Can you work these out from the model? Positions are in its coordinate system, mm. A direction names the side the tool comes from. Round coordinates to 2 decimals unless told otherwise and drop trailing zeros. Order: outer loops, then holes, each group sorted by start corner. A loop starts at its lowest first (then second) coordinate and runs counter-clockwise, first axis right, second up.
Q1. For faces 5 (the face through (18.288, -19, 13)), 6 (the face through (105, -20.32, 13)), which set-ups out of +Z, -Z, +X, -X, +Y, -Y let a thin tool reach every point of the face, with its end or its side?
Q2. If we section it at A-A (y = -14): Count the separate pieces of the cut face and the enclosed holes in it, plus the area to 3 significant figures.
Q3. If we section it at C-C (x = 53.5): Please give me the cut outline in (y, z).
Q4. Will this pin go through, and if not, where does the flat tip stop? P1, Ø10, axis at x = 89, z = 21, coming from the -Y side.
Q5. If I drill on line 1 (X direction, y = -15.75, z = 7.5); line 2 (X direction, y = -13.5, z = 14.75); line 3 (Y direction, x = 55, z = 6.75), over which ranges is the centre line in solid material (lowest first)?
Q6. We'd pull the mould along X, two halves only. Please class faces 1 (the face through (58, -8, 25.4)), 2 (the face through (33.25, -16.51, 12.52)), 3 (the face through (96.012, -19, 13)), 4 (the face through (114.3, -10, 13)): pulls with the +X half, pulls with the -X half, needs draft (parallel to the pull), parting line crosses it, or undercut.
Q7. If we section it at B-B (x = 71): Please give me the cut outline in (y, z).
from build123d import *

# Parameters (mm, degrees)
F1_DEPTH = 25.4


with BuildPart() as f1:
    # F0 (on Top) → F1 (new body)
    with BuildSketch(Plane.XY):
        with BuildLine():
            Line((57.15, 0), (0, 0))
            Line((0, 0), (0, -20.32))
            Line((0, -20.32), (18.288, -20.32))
            Line((18.288, -20.32), (18.288, -17.78))
            add(Edge.make_bspline(
                [(18.288, -17.78), (19.5003372633, -17.78), (20.9589545485, -17.4917433662), (23.0646434791, -15.3048474183), (24.9900381466, -13.3300613523), (27.3662145743, -12.7), (28.575, -12.7)],
                knots=[0, 0, 0, 0, 0.2397485597, 0.4832453932, 0.7259444723, 1, 1, 1, 1], degree=3))
            ThreePointArc((28.575, -12.7), (33.3375, -16.51), (38.1, -12.7))
            ThreePointArc((38.1, -12.7), (47.2236683009, -16.8621762468), (57.15, -18.288))
            Line((57.15, -18.288), (57.15, 0))
        make_face()
    extrude(amount=F1_DEPTH)

    # F2: F1 across face


with BuildPart() as f1_1:
    add(f1.part)
    add(f1.part.mirror(Plane(origin=(57.15, -9.144, 12.7), x_dir=(0, 1, 0), z_dir=(1, 0, 0))))


solid = f1_1.part
Solution:
1. face 5: +Z, -Z, -Y
1. face 6: +Z, -Z, +X, -X, -Y
2. separate pieces: 5
2. enclosed holes: 0
2. area: 2,530 mm2
3. outline: (-18.1, 0) - (0, 0) - (0, 25.4) - (-18.1, 25.4) - close
4. P1: stops at y = -17.51
5. line 1: x = 0 to 22.64, 30.72 to 35.95, 44.01 to 70.29, 78.35 to 83.58, 91.66 to 114.3
5. line 2: x = 0 to 25.27, 28.83 to 37.85, 39.41 to 74.89, 76.45 to 85.47, 89.03 to 114.3
5. line 3: y = -18.22 to 0
6. face 1: needs draft
6. face 2: undercut
6. face 3: undercut
6. face 4: pulls with the +X half
7. outline: (-15.45, 0) - (0, 0) - (0, 25.4) - (-15.45, 25.4) - close
